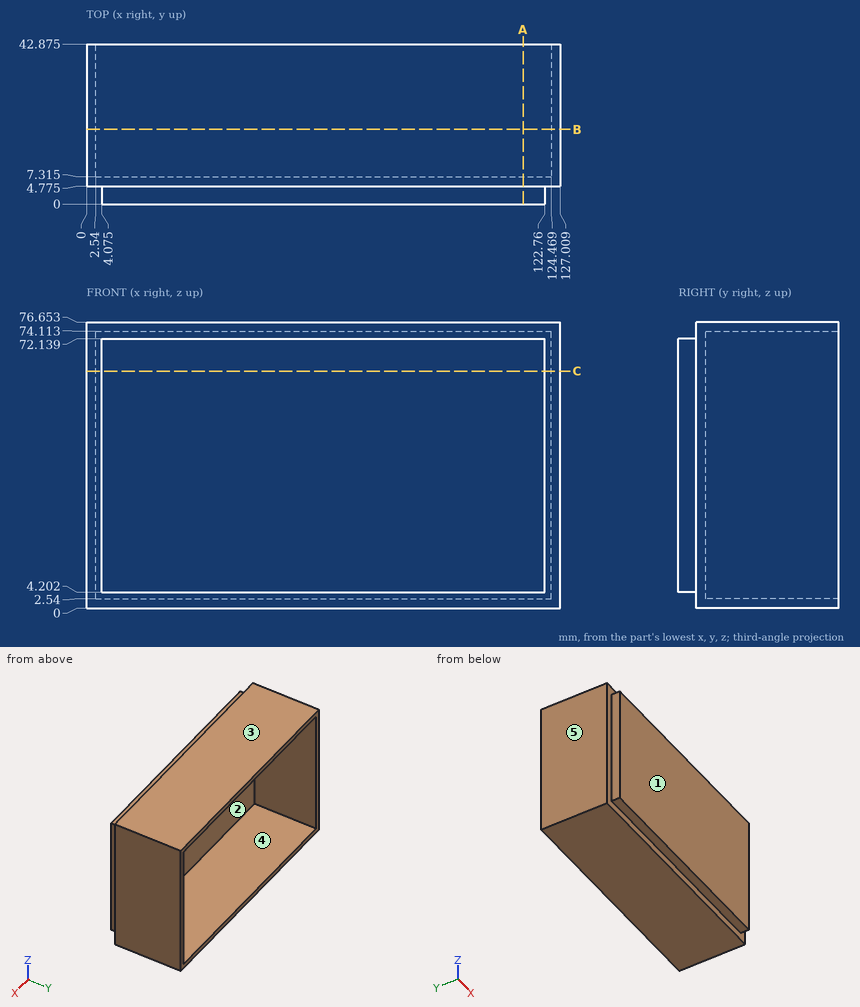
Geometry check sheet. Reference: drawing and pictorial views, mm from the part's lowest x, y, z. A direction names the side the tool comes from. Give positions to 0.01 mm unless a question says otherwise; leave off trailing zeros. Write each loop counter-clockwise with the first axis right and the second up, starting at its lowest first coordinate (ties: lowest second). Pieces come first, ordered by that corner, then holes. Notation, with made-up numbers: (-30.5, 69) -> (21.5, 69) arc R17 ccw to (21.5, 102) -> close; hole circle Ø1 at (55.5, 22.5). An arc over 180 degrees is marked (long way). One line per question, with ' | ' between items.
Item 1: Sectioned sample at A-A, the plane x = 117. Record the boundary of the cut face in (y, z) (1 decimal), plus the area to 3 significant figures.
Determined:
outline: (0, 4.2) -> (4.8, 4.2) -> (4.8, 0) -> (42.9, 0) -> (42.9, 2.5) -> (7.3, 2.5) -> (7.3, 74.1) -> (42.9, 74.1) -> (42.9, 76.7) -> (4.8, 76.7) -> (4.8, 72.1) -> (0, 72.1) -> close | area: 700 mm^2
Item 2: Draft check along Z on the marked faces 1, 2 and 3. Enter one of: released by +Z, released by -Z, zero draft, split by the parting line, or undercut.
Determined:
face 1: zero draft | face 2: undercut | face 3: released by +Z
Item 3: Scan lines: line 1 along Z through (x, y) = (70, 15); line 2 along X through (y, z) = (30, 48); line 3 along Y through (x, z) = (31.5, 53) (1 decimal). Record each from-to range of solid material in increasing order.
Determined:
line 1: 0 to 2.54, 74.11 to 76.65 | line 2: 0 to 2.54, 124.47 to 127.01 | line 3: 0 to 7.3
Item 4: Access from +Z, -Z, +X, -X, +Y, -Y to the whole of each face (thin tool, end or side, straight path). Record for the marked faces 4 and 5.
Determined:
face 4: +Y | face 5: +Z, -Z, -X, +Y, -Y
Item 5: Depth check by flat-ended pin: pin 1 (23 mm diameter, centred on x = 67.5, z = 52.5, fed in from -Y). Enter the tip coordinate at first touch or a pass-through.
Determined:
pin 1: y = 0
Item 6: Sectioned sample at C-C, the plane z = 63.5. Record the boundary of the cut face in (x, y) (1 decimal), plus the area to 3 significant figures.
Determined:
outline: (0, 4.8) -> (4.1, 4.8) -> (4.1, 0) -> (122.8, 0) -> (122.8, 4.8) -> (127, 4.8) -> (127, 42.9) -> (124.5, 42.9) -> (124.5, 7.3) -> (2.5, 7.3) -> (2.5, 42.9) -> (0, 42.9) -> close | area: 1,070 mm^2
Item 7: Sectioned sample at B-B, the plane y = 20. Record the boundary of the cut face in (x, z), plus the area to 3 significant figures.
Determined:
outline: (0, 0) -> (127.01, 0) -> (127.01, 76.65) -> (0, 76.65) -> close; hole (2.54, 2.54) -> (124.47, 2.54) -> (124.47, 74.11) -> (2.54, 74.11) -> close | area: 1,010 mm^2
